Read the model definition and answer for the solid it produces. Units are mm, in the model's axes. A direction names the side the tool comes from. Coordinates: 2 decimals unless noted, no trailing zeros. Loops run counter-clockwise (first coordinate to the right, second up) from the corner with the lowest first, then second, coordinate; pieces in that order, holes last.
Q1. The mould has two halves that part along Y. Classify faces 1 (the face through (-3, -20, 0)), 2 (the face through (0, 5, 6)), 3 (the face through (9.46, -2.3, -20.39)), 4 (the face through (-3, 20, 0)): pulls with the +Y half, pulls with the -Y half, needs draft (parallel to the pull), parting line crosses it, or undercut.
Q2. Section B-B (y = 0) is taken. Give the vertices of the cut face in (x, z), then the cut area to 4 significant figures.
Q3. Section C-C (z = 24) is taken. Give the vertices of the cut face in (x, y).
Q4. Which of the six approach directions +Z, -Z, +X, -X, +Y, -Y give full straight-line access (tool end or side, diameter ignored) to faces 5 (the face through (8, 0, -13)), 6 (the face through (8, 0, -28))?
Q5. A flat-ended cylindrical pin translates along its axis: P1, Ø24, axis at y = 0, z = 0, coming from the +X side. Find the tip coordinate at first contact, or state that the pin passes through.
Q6. Straight lines are drawn through the part: line 1 (Y direction, x = -8, z = 0); line 2 (Z direction, x = 22, y = -0.5); line 3 (X direction, y = 0, z = 24). For each, find the intervals that lie inside material, in ascending order.
Q7. Section A-A (x = 22) is taken. Give the vertices of the cut face in (y, z), then the cut area to 3 significant figures.
Q8. Section D-D (x = 15) is taken. Give the vertices of the cut face in (y, z).
from build123d import *

# Parameters (mm, degrees)
SKETCH1_W               = 15
SKETCH1_H               = 40
SKETCH1_W_2             = 26
SKETCH1_R               = 7.5
BOSS_EXTRUDE1_DEPTH     = 15
SKETCH1_3_W             = 15
SKETCH1_3_H             = 40
BOSS_EXTRUDE2_DEPTH     = 30
CUT_EXTRUDE1_DEPTH      = 55.598534779
CUT_EXTRUDE1_DEPTH_BACK = 55.598534779
SKETCH2_R               = 6


with BuildPart() as part:
    # Sketch1 → Boss-Extrude1 (new body)
    # profile 1 of 3: a face of its own
    with BuildSketch(Plane(origin=(0, 0, 0), x_dir=(0, 0, -1), z_dir=(1, 0, 0))):
        with Locations((-20.5, 0)):
            Rectangle(SKETCH1_W, SKETCH1_H)
    # profile 2 of 3: a face of its own
    with BuildSketch(Plane(origin=(0, 0, 0), x_dir=(0, 0, -1), z_dir=(1, 0, 0))):
        Rectangle(SKETCH1_W_2, SKETCH1_H)
        Circle(SKETCH1_R, mode=Mode.SUBTRACT)
    # profile 3 of 3: a face of its own
    with BuildSketch(Plane(origin=(0, 0, 0), x_dir=(0, 0, -1), z_dir=(1, 0, 0))):
        with Locations((20.5, 0)):
            Rectangle(SKETCH1_W, SKETCH1_H)
    extrude(amount=-BOSS_EXTRUDE1_DEPTH)

    # Sketch1_3 → Boss-Extrude2 (add)
    with BuildSketch(Plane(origin=(0, 0, 0), x_dir=(0, 0, -1), z_dir=(1, 0, 0))):
        with Locations((-20.5, 0)):
            Rectangle(SKETCH1_3_W, SKETCH1_3_H)
        with Locations((20.5, 0)):
            Rectangle(SKETCH1_3_W, SKETCH1_3_H)
    extrude(amount=BOSS_EXTRUDE2_DEPTH)

    # Sketch2 → Cut-Extrude1 (cut, two sides: drawn at the far end of the back side and taken through both)
    with BuildSketch(Plane(origin=(0, 0, 13), x_dir=(-1, 0, 0), z_dir=(0, 0, -1)).offset(-CUT_EXTRUDE1_DEPTH_BACK)):
        with Locations((-15, 0)):
            Circle(SKETCH2_R)
    extrude(amount=CUT_EXTRUDE1_DEPTH + CUT_EXTRUDE1_DEPTH_BACK, mode=Mode.SUBTRACT)


solid = part.part
Numbers:
1. face 1: pulls with the -Y half
1. face 2: needs draft
1. face 3: undercut
1. face 4: pulls with the +Y half
2. outline: (-15, -28) - (9, -28) - (9, -13) - (0, -13) - (0, -7.5) - (-15, -7.5) - close; (-15, 7.5) - (0, 7.5) - (0, 13) - (9, 13) - (9, 28) - (-15, 28) - close; (21, -28) - (30, -28) - (30, -13) - (21, -13) - close; (21, 13) - (30, 13) - (30, 28) - (21, 28) - close
2. area: 1,155 mm2
3. outline: (-15, -20) - (30, -20) - (30, 20) - (-15, 20) - close; hole circle Ø12 at (15, 0)
4. face 5: +X, +Y, -Y
4. face 6: -Z, +X, -X, +Y, -Y
5. P1: stops at x = 0
6. line 1: y = -20 to -7.5, 7.5 to 20
6. line 2: z = -28 to -13, 13 to 28
6. line 3: x = -15 to 9, 21 to 30
7. outline: (-20, -28) - (20, -28) - (20, -13) - (-20, -13) - close; (-20, 13) - (20, 13) - (20, 28) - (-20, 28) - close
7. area: 1,200 mm2
8. outline: (-20, -28) - (-6, -28) - (-6, -13) - (-20, -13) - close; (-20, 13) - (-6, 13) - (-6, 28) - (-20, 28) - close; (6, -28) - (20, -28) - (20, -13) - (6, -13) - close; (6, 13) - (20, 13) - (20, 28) - (6, 28) - close
